Geometry: final body of the model. Coordinates: model frame, mm. Round coordinates to 2 decimals unless told otherwise and drop trailing zeros. Loops run counter-clockwise (first coordinate to the right, second up) from the corner with the lowest first, then second, coordinate; pieces in that order, holes last. Notation, with made-up numbers: (-39.5, 3.5) -> (-14.5, 3.5) arc R20 cw to (-14.5, 36.5) -> close; hole circle Ø6 at (-34.75, 13.5). An arc over 180 degrees is marked (long way). Answer in a Markdown table with one row per item.
```python
from build123d import *

# Parameters (mm, degrees)
SKETCH1_R           = 1.5875
BOSS_EXTRUDE1_DEPTH = 120.65
SKETCH3_R           = 1.5875
BOSS_EXTRUDE2_DEPTH = 125.4125
LPATTERN1_COUNT     = 6
LPATTERN1_PITCH     = 47.625


with BuildPart() as part:
    # Sketch1 → Boss-Extrude1 (new body, symmetric)
    with BuildSketch(Plane(origin=(0, 0, 0), x_dir=(0, 0, -1), z_dir=(1, 0, 0))):
        Circle(SKETCH1_R)
    extrude(amount=BOSS_EXTRUDE1_DEPTH, both=True)

    # Sketch3 → Boss-Extrude2 (add)
    with BuildSketch(Plane.XY):
        with Locations((-119.0625, 0)):
            Circle(SKETCH3_R)
    boss_extrude2 = extrude(amount=BOSS_EXTRUDE2_DEPTH)

    # LPattern1: Boss-Extrude2 ×6
    with Locations(*[(i * LPATTERN1_PITCH, 0, 0) for i in range(1, LPATTERN1_COUNT)]):
        add(boss_extrude2)


solid = part.part
```
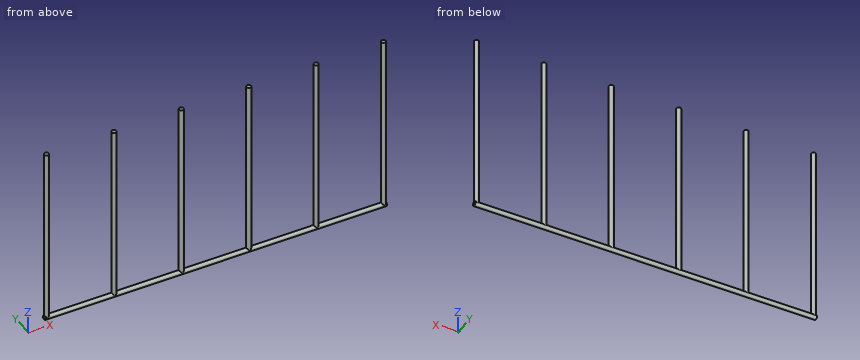
Item 1: Section query C-C, the plane x = -16.5. Output: boundary loops of the cut face in (y, z) (1 decimal).
Ans:
| item | result |
|---|---|
| outline | circle Ø3.2 at (0, 0) |
Item 2: Section query B-B, the plane y = 0.95. Output: boundary loops of the cut face in (x, z), and give its area (3 significant figures).
Ans:
| item | result |
|---|---|
| outline | (-120.65, -1.27) -> (120.65, -1.27) -> (120.65, 1.27) -> (120.33, 1.27) -> (120.33, 125.41) -> (117.79, 125.41) -> (117.79, 1.27) -> (72.71, 1.27) -> (72.71, 125.41) -> (70.17, 125.41) -> (70.17, 1.27) -> (25.08, 1.27) -> (25.08, 125.41) -> (22.54, 125.41) -> (22.54, 1.27) -> (-22.54, 1.27) -> (-22.54, 125.41) -> (-25.08, 125.41) -> (-25.08, 1.27) -> (-70.17, 1.27) -> (-70.17, 125.41) -> (-72.71, 125.41) -> (-72.71, 1.27) -> (-117.79, 1.27) -> (-117.79, 125.41) -> (-120.33, 125.41) -> (-120.33, 1.27) -> (-120.65, 1.27) -> close |
| area | 2,510 mm2 |
Item 3: Section query A-A, the plane z = 17. State how many separate pieces and enclosed holes the cut face has, and give its area (3 significant figures).
Ans:
| item | result |
|---|---|
| separate pieces | 6 |
| enclosed holes | 0 |
| area | 47.5 mm2 |
Item 4: Ray query, L1, parallel to X at y = -0.4, z = 86; L2, parallel to X at y = 0.2, z = 13; L3, parallel to Z at x = 50, y = 0.4. Return the intervals inside material, ascending.
Ans:
| item | result |
|---|---|
| L1 | -120.6 to -117.53, -72.97 to -69.9, -25.35 to -22.28, 22.28 to 25.35, 69.9 to 72.97, 117.53 to 120.6 |
| L2 | -120.64 to -117.49, -73.01 to -69.86, -25.39 to -22.24, 22.24 to 25.39, 69.86 to 73.01, 117.49 to 120.64 |
| L3 | -1.54 to 1.54 |
Item 5: First-contact query: P1, Ø1.5, axis at x = -22, z = 94, coming from the -Y side. Flat tip, straight axial feed; report the tip coordinate or a pass-through.
Ans:
| item | result |
|---|---|
| P1 | y = -1.18 |
